Verification items for the finished model (mm, model axes). A direction names the side the tool comes from. Coordinates: 2 decimals unless noted, no trailing zeros. Loops run counter-clockwise (first coordinate to the right, second up) from the corner with the lowest first, then second, coordinate; pieces in that order, holes last. Notation, with made-up numbers: (-6, 84) - (19, 84) arc R8 cw to (19, 93) - close; hole circle Ø11 at (-17, 67.5). An arc over 180 degrees is marked (long way). One line per item, written item: value. Start each with the question number.
(1) Section check A-A (z = 0). Record the boundary of the cut face in (x, y), plus the area to 3 significant figures.
(2) Draft check along Y on faces 1 (the face through (0, -3, 11)), 2 (the face through (28, -25, 11)), 3 (the face through (24.65, 10.635, -3.349)), 4 (the face through (24.65, 11.777, -3.709)). Enter one of: +Y half, -Y half, draft (parallel to the pull), parting line (faces both ways), or undercut.
(3) Gauge pin test, flat ends, axial feed: P1, Ø8, axis at y = -16, z = -6, coming from the -X side; P2, Ø1.5, axis at y = -8.5, z = 0.5, coming from the +X side; P3, Ø3, axis at x = 8, z = -7.5, coming from the -Y side; P4, Ø5, axis at x = 30.5, y = -17.5, coming from the +Z side. Record the tip position at first contact, or that the pin passes through.
(4) Thickness scan on probe 1 along Y at (x, z) = (6, -0.5); probe 2 along Z at (x, y) = (25, -13.5); probe 3 along Y at (x, z) = (33, 0). Record the ranges inside material, lowest first. Write a range as [from, to].
(5) Set-up check for faces 5 (the face through (50, -3, 11)), 6 (the face through (37.336, -15.453, -0.543)): record each of +Z, -Z, +X, -X, +Y, -Y from which the full face is reachable in a straight line by a thin tool's end or side.
Autodesk Inventor part; units mm, degrees
ref_plane "Work Plane2" through (0, -25, 0) normal (0, 1, 0) x (-1, 0, 0)
ref_plane "YZ Plane" through (0, 0, 0) normal (1, 0, 0) x (0, 1, 0)
ref_plane "XY Plane" through (0, 0, 0) normal (0, 0, 1) x (1, 0, 0)
sketch "Sketch1" plane through (0, 0, 0) normal (1, 0, 0) x (0, 1, 0)
  circle A0 centre (0, 0) radius 11.15
  circle A1 centre (0, 0) radius 12.3475
  dimension "d0" = 22.3
  dimension "d1" = 24.695
extrude "Extrusion1" add sketch "Sketch1" along normal blind 50
ref_plane "Work Plane2" through (0, -25, 0) normal (0, 1, 0) x (-1, 0, 0)
sketch "Sketch2" plane through (0, -25, 0) normal (0, 1, 0) x (-1, 0, 0)
  line L0 (0, 0) -> (-50, 0)
  line L1 (-50, 12.3475) -> (-50, -12.3475)
  circle A0 centre (-25, 0) radius 12.3475
  circle A1 centre (-25, 0) radius 11.15
  dimension "d6" = 50
  dimension "d7" = 22.3
extrude "Extrusion2" add sketch "Sketch2" along normal blind 25 contours A0 L0 A1 | L0 A1 A0
sketch "Sketch3" plane through (0, 0, 0) normal (-1, 0, 0) x (0, 0, 1)
  line L0 (11.15, 0) -> (-11.15, 0)
  circle A0 centre (0, 0) radius 11.15
extrude "Extrusion3" cut sketch "Sketch3" against normal blind 78.975
sketch "Sketch4" plane through (25, -25, 0) normal (0, -1, 0) x (1, 0, 0)
  circle A0 centre (0, 0) radius 11.15
  point P0 (-25, 0)
extrude "Extrusion4" cut sketch "Sketch4" against normal blind 25
properties part number "Connector" material "PVC-Piping"
Responses:
1. outline: (0, -12.35) - (12.65, -12.35) - (12.65, -25) - (13.85, -25) - (13.85, -11.15) - (0, -11.15) - close; (0, 11.15) - (50, 11.15) - (50, 12.35) - (0, 12.35) - close; (36.15, -25) - (37.35, -25) - (37.35, -12.35) - (50, -12.35) - (50, -11.15) - (36.15, -11.15) - close
1. area: 123 mm²
2. face 1: draft
2. face 2: -Y half
2. face 3: undercut
2. face 4: parting line
3. P1: stops at x = 12.82
3. P2: passes through
3. P3: stops at y = -10.79
3. P4: stops at z = 11.98
4. probe 1: y = [-12.34, -11.14], [11.14, 12.34]
4. probe 2: z = [-12.35, -11.15], [11.15, 12.35]
4. probe 3: y = [11.15, 12.35]
5. face 5: +Z, -Z, +X, +Y, -Y
5. face 6: -Y
